Check sheet for the drawn part. Datum: minimum x, y, z corner. Units: mm. A direction names the side the tool comes from. Round coordinates to 2 decimals unless told otherwise and drop trailing zeros. Write each loop counter-clockwise with the first axis right and the second up, starting at its lowest first coordinate (ties: lowest second). Pieces come first, ordered by that corner, then holes. Notation, with made-up numbers: M 26.5,-28.5 L 52.5,-28.5 A8 cw 52.5,-24.5 Z; hole C -34,80 d8. An arc over 180 degrees is marked long. One line per item, written item: value.
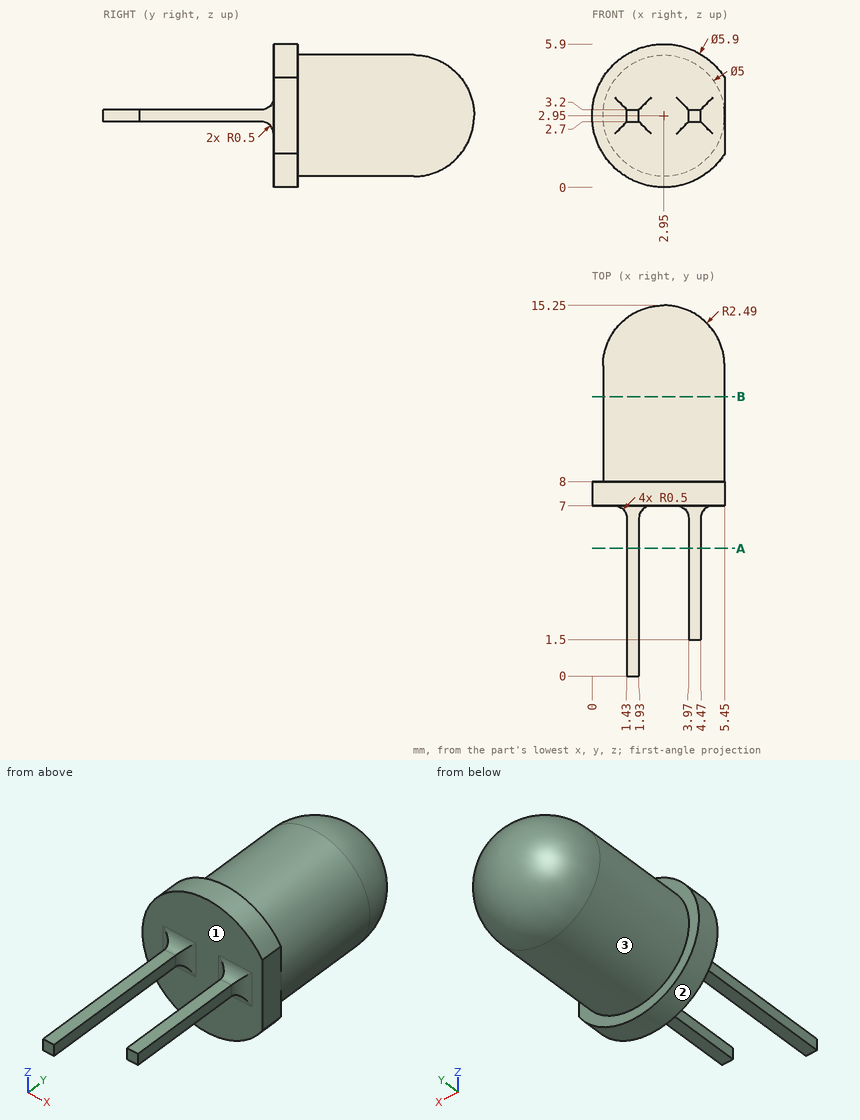
Q1. Sectioned sample at B-B on y = 11.5. Enter the section's corners in (x, z), and give its area (3 significant figures).
Completed:
outline: C 2.95,2.95 d5
area: 19.6 mm^2
Q2. Access from +Z, -Z, +X, -X, +Y, -Y to the whole of each face (thin tool, end or side, straight path). Record for the marked faces 1, 2 and 3.
Completed:
face 1: -Y
face 2: +Y, -Y
face 3: +Y
Q3. Scan lines: line 1 (Y direction, x = 0.65, z = 4.05); line 2 (X direction, y = 10.5, z = 1) (1 decimal); line 3 (Z direction, x = 2.6, y = 7.75). Record each from-to range of solid material in increasing order. Write a range as [from, to].
Completed:
line 1: [7, 8]
line 2: [1.4, 4.5]
line 3: [0.02, 5.88]
Q4. Depth check by flat-ended pin: P1, Ø1, axis at x = 4.5, y = 2.5, coming from the -Z side; P2, Ø1, axis at x = 4.5, z = 2.5, coming from the +Y side; P3, Ø1, axis at x = 0.5, y = 8, coming from the -Z side. Enter the tip coordinate at first touch or a pass-through.
Completed:
P1: z = 2.7
P2: y = 14.99
P3: z = 0.74
Q5. Sectioned sample at A-A on y = 5.25. Enter the section's corners in (x, z).
Completed:
outline: M 1.43,2.7 L 1.93,2.7 L 1.93,3.2 L 1.43,3.2 Z; M 3.97,2.7 L 4.47,2.7 L 4.47,3.2 L 3.97,3.2 Z
